Answer from the drawing. Dimensions are ordinates in mm from the lowest x, y and z of the part. A direction names the side the tool comes from. Give positions to 0.01 mm unless a question says otherwise; leave off trailing zeros. Write each loop counter-clockwise with the first axis right and the second up, starting at its lowest first coordinate (ties: lowest second). Pieces come first, ordered by that corner, then holes. Notation, with made-up numbers: (64.25, 22.5) -> (75.25, 22.5) arc R9 ccw to (75.25, 33.5) -> close; hole circle Ø9 at (14, -23). An arc over 180 degrees is marked (long way). Write item = value, one per line.
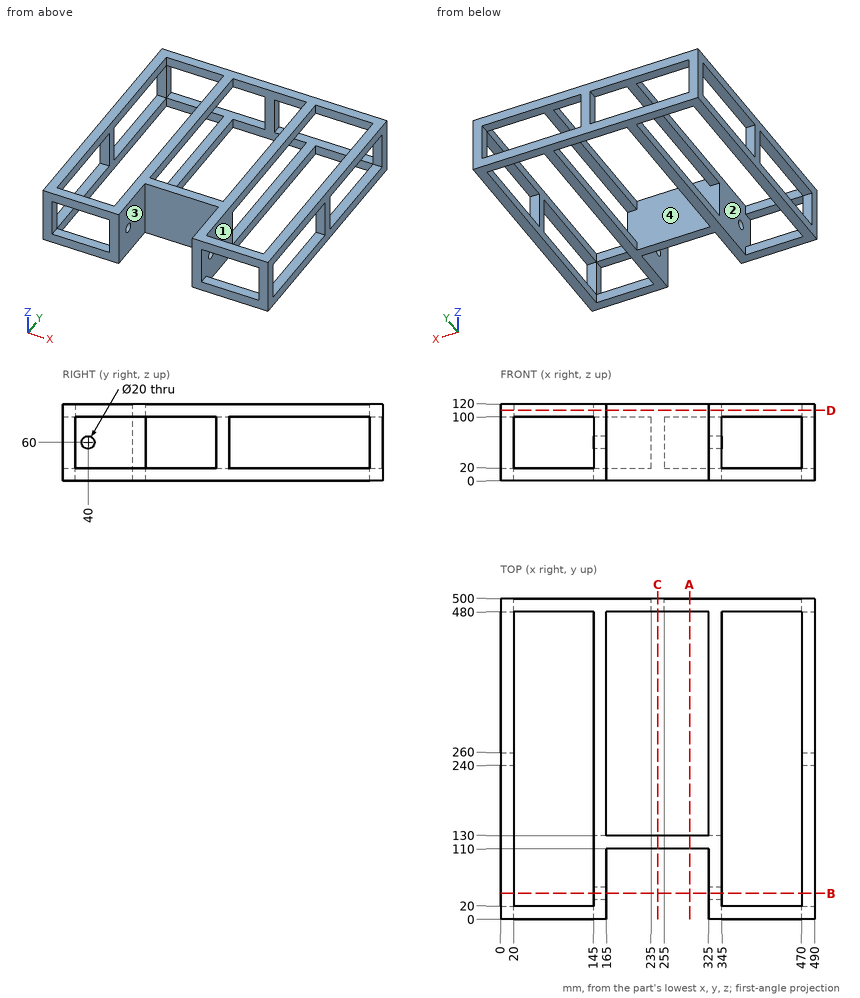
(1) For a pull along X with two mould halves and no side action, classify the marked faces 1 and 2 as released by +X, released by -X, zero draft, split by the parting line, or undercut.
Checks:
face_1 = undercut
face_2 = undercut
(2) Given P1, Ø1, axis at y = 56.5, z = 56.5, coming from the -X side, flat-ended and moving along its own axis, determine where the tip first touches the part or whether it passes through.
Checks:
P1 = 145
(3) A tool of negligible diameter and unlimited length cuts with its end or side. For the marked faces 3 and 4, from which of +Z, -Z, +X, -X, +Y, -Y can it reach the whole face along a straight path? Write none if from no direction.
Checks:
face_3 = +Z, -Z, -Y
face_4 = none
(4) The part is cut by section D-D on z = 110. Determine the outline of the cut face in (x, y), plus the area to 3 significant figures.
Checks:
outline = (0, 0) -> (165, 0) -> (165, 110) -> (325, 110) -> (325, 0) -> (490, 0) -> (490, 500) -> (0, 500) -> close; hole (20, 20) -> (145, 20) -> (145, 480) -> (20, 480) -> close; hole (165, 130) -> (325, 130) -> (325, 480) -> (165, 480) -> close; hole (345, 20) -> (470, 20) -> (470, 480) -> (345, 480) -> close
area = 56,400 mm²
(5) The part is cut by section A-A on x = 295. Determine the outline of the cut face in (y, z), plus the area to 3 significant figures.
Checks:
outline = (110, 0) -> (130, 0) -> (130, 120) -> (110, 120) -> close; (480, 0) -> (500, 0) -> (500, 20) -> (480, 20) -> close; (480, 100) -> (500, 100) -> (500, 120) -> (480, 120) -> close
area = 3,200 mm²
(6) The part is cut by section C-C on x = 245. Determine the outline of the cut face in (y, z), plus the area to 3 significant figures.
Checks:
outline = (110, 0) -> (130, 0) -> (130, 120) -> (110, 120) -> close; (480, 0) -> (500, 0) -> (500, 120) -> (480, 120) -> close
area = 4,800 mm²
(7) Consider L1, parallel to X at y = 276.5, z = 7; L2, parallel to Z at x = 340, y = 40; L3, parallel to Y at x = 200.5, z = 14. Determine where each line is inside the solid, lowest interval first.
Checks:
L1 = 0 to 20, 145 to 165, 325 to 345, 470 to 490
L2 = 0 to 50, 70 to 120
L3 = 110 to 130, 480 to 500
(8) The part is cut by section B-B on y = 40. Count the separate pieces of the cut face and the enclosed holes in it, plus the area to 3 significant figures.
Checks:
separate_pieces = 8
enclosed_holes = 0
area = 5,600 mm²
